Build history of the part. All positions in model axes, mm. A direction names the side the tool comes from. Round coordinates to 2 decimals unless told otherwise and drop trailing zeros. Loops run counter-clockwise (first coordinate to the right, second up) from the corner with the lowest first, then second, coordinate; pieces in that order, holes last. Notation, with made-up numbers: (-23, -19) - (-13, -19) arc R5 cw to (-13, -10) - close; hole circle Ø5 at (-30, 53.5). An arc over 180 degrees is marked (long way). Use a Markdown table: item, result.
from build123d import *

# Parameters (mm, degrees)
SKETCH1_R           = 3.34
BOSS_EXTRUDE1_DEPTH = 4.913831128
SKETCH1_3_R         = 3.34
BOSS_EXTRUDE2_DEPTH = 61


with BuildPart() as part:
    # Sketch1 → Boss-Extrude1 (new body)
    # profile 1 of 2: a face of its own
    with BuildSketch(Plane(origin=(0, 0, 0), x_dir=(0, 0, -1), z_dir=(1, 0, 0))):
        Polygon((-8.000668903, -0.149990369), (-3.870438982, -7.003777701), (4.130229921, -6.853787333), (8.000668903, 0.149990369), (3.870438982, 7.003777701), (-4.130229921, 6.853787333), align=None)
        Circle(SKETCH1_R, mode=Mode.SUBTRACT)
    # profile 2 of 2: a face of its own
    with BuildSketch(Plane(origin=(0, 0, 0), x_dir=(0, 0, -1), z_dir=(1, 0, 0))):
        Circle(SKETCH1_R)
    extrude(amount=BOSS_EXTRUDE1_DEPTH)

    # Sketch1_3 → Boss-Extrude2 (add)
    with BuildSketch(Plane(origin=(0, 0, 0), x_dir=(0, 0, -1), z_dir=(1, 0, 0))):
        with Locations(Location((0, 0, 0), (0, 0, 180))):
            Circle(SKETCH1_3_R)
    extrude(amount=BOSS_EXTRUDE2_DEPTH)


solid = part.part
Q1. Cut at B-B, the plane x = 8. List the corners of the cut face in (y, z), plus the area to 3 significant figures.
Results found:
| item | result |
|---|---|
| outline | circle Ø6.68 at (0, 0) |
| area | 35.0 mm2 |
Q2. Drop flat-ended pins along their axis: pin 1 (6 mm diameter, centred on x = 50, y = 1.5, fed in from -Z); pin 2 (8 mm diameter, centred on x = 30.5, y = -1, fed in from +Z); pin 3 (5 mm diameter, centred on x = 33.5, z = -3, fed in from -Y); pin 4 (1 mm diameter, centred on x = 11.5, z = 4.5, fed in from +Y). Give the stop position or say it passes through.
Results found:
| item | result |
|---|---|
| pin 1 | stops at z = -3.34 |
| pin 2 | stops at z = 3.34 |
| pin 3 | stops at y = -3.3 |
| pin 4 | passes through |
Q3. Cut at A-A, the plane z = 0. List the corners of the cut face in (x, y).
Results found:
| item | result |
|---|---|
| outline | (0, -6.93) - (4.91, -6.93) - (4.91, -3.34) - (61, -3.34) - (61, 3.34) - (4.91, 3.34) - (4.91, 6.93) - (0, 6.93) - close |
Q4. Pull direction X, two halves, no side cores. Call faces 3 (the face through (4.914, -3, -2)), 4 (the face through (0, 0, 0)), 5 (the face through (2.423, 3.529, -5.964)): pulls with the +X half, pulls with the -X half, needs draft (parallel to the pull), parting line crosses it, or undercut.
Results found:
| item | result |
|---|---|
| face 3 | pulls with the +X half |
| face 4 | pulls with the -X half |
| face 5 | needs draft |
Q5. Which spindle directions (+Z, -Z, +X, -X, +Y, -Y) get a long thin tool onto all of the face, cutting with end or side? Do faces 1 (the face through (61, 0, 0)), 2 (the face through (32.56, 3.26, -0.72)). Say none if no direction does.
Results found:
| item | result |
|---|---|
| face 1 | +Z, -Z, +X, +Y, -Y |
| face 2 | +X |
Q6. Probe line 1 (X direction, y = 6.25, z = 3.75); line 2 (Z direction, x = 28.5, y = 1.25); line 3 (Y direction, x = 49.5, z = -0.5). List the from-to ranges inside material, lowest first.
Results found:
| item | result |
|---|---|
| line 1 | x = 0 to 4.91 |
| line 2 | z = -3.1 to 3.1 |
| line 3 | y = -3.3 to 3.3 |
Q7. Cut at C-C, the plane y = -4. List the corners of the cut face in (x, z).
Results found:
| item | result |
|---|---|
| outline | (0, -5.71) - (4.91, -5.71) - (4.91, 5.68) - (0, 5.68) - close |
Q8. Cut at D-D, the plane z = -2.5. List the corners of the cut face in (x, y), plus the area to 3 significant figures.
Results found:
| item | result |
|---|---|
| outline | (0, -6.88) - (4.91, -6.88) - (4.91, -2.21) - (61, -2.21) - (61, 2.21) - (4.91, 2.21) - (4.91, 6.98) - (0, 6.98) - close |
| area | 317 mm2 |
